from build123d import *

# Parameters (mm, degrees)
SKETCH3_R               = 3
CUT_EXTRUDE1_DEPTH      = 75.457245764
SKETCH4_R               = 41.3
SKETCH4_R_2             = 38
SKETCH4_R_3             = 3
CUT_EXTRUDE2_DEPTH      = 10
BOSS_EXTRUDE1_START     = -2
BOSS_EXTRUDE1_OUTLINE_R = 41.3
BOSS_EXTRUDE1_DEPTH     = 2
SKETCH5_R               = 3
SKETCH5_R_2             = 1.7
BOSS_EXTRUDE2_DEPTH     = 2


# Read off the part's stored shape, not the designer's step: Boss-Extrude1
with BuildPart() as part:
    # Sketch2 → Revolve1 (revolve)
    with BuildSketch(Plane(origin=(0, 0, 0), x_dir=(1, 0, 0), z_dir=(0, 1, 0)), mode=Mode.PRIVATE) as revolve1_sk:
        Polygon((-21.165551628, 4), (-21.165551628, -4), (-9.945763659, -4), align=None)
    revolve(revolve1_sk.sketch.rotate(Axis((20.134448372, 0, 4), (0, 0, -1)), 180), axis=Axis((20.134448372, 0, 4), (0, 0, -1)))

    # Sketch3 → Cut-Extrude1 (cut, through all)
    with BuildSketch(Plane.XY.offset(4)):
        with Locations((20.134448372, 35.5)):
            Circle(SKETCH3_R)
        with Locations((55.634448372, 0)):
            Circle(SKETCH3_R)
        with Locations((20.134448372, -35.5)):
            Circle(SKETCH3_R)
        with Locations((-15.365551628, 0)):
            Circle(SKETCH3_R)
    extrude(amount=-CUT_EXTRUDE1_DEPTH, mode=Mode.SUBTRACT)

    # Sketch4 → Cut-Extrude2 (cut)
    # profile 1 of 4: a face of its own
    with BuildSketch(Plane.XY.offset(4)):
        with Locations((20.134448372, 0)):
            Circle(SKETCH4_R)
        with Locations((20.134448372, 0)):
            Circle(SKETCH4_R_2, mode=Mode.SUBTRACT)
        with Locations((55.634448372, 0)):
            Circle(SKETCH4_R_3, mode=Mode.SUBTRACT)
    # profile 2 of 4: a face of its own
    with BuildSketch(Plane.XY.offset(4)):
        with Locations((20.134448372, -35.5)):
            Circle(SKETCH4_R_3)
    # profile 3 of 4: a face of its own
    with BuildSketch(Plane.XY.offset(4)):
        with Locations((-15.365551628, 0)):
            Circle(SKETCH4_R_3)
    # profile 4 of 4: a face of its own
    with BuildSketch(Plane.XY.offset(4)):
        with Locations((20.134448372, 35.5)):
            Circle(SKETCH4_R_3)
    extrude(amount=-CUT_EXTRUDE2_DEPTH, mode=Mode.SUBTRACT)

    # Boss-Extrude1 outline → Boss-Extrude1 (add)
    with BuildSketch(Plane.XY.offset(4).offset(BOSS_EXTRUDE1_START)):
        with Locations((20.134448372, 0)):
            Circle(BOSS_EXTRUDE1_OUTLINE_R)
        with BuildLine():
            ThreePointArc((21.849721462, 37.961267606), (47.004506057, 26.870057685), (58.095715978, 1.71527309))
            ThreePointArc((58.095715978, 1.71527309), (58.634448372, 0), (58.095715978, -1.71527309))
            ThreePointArc((58.095715978, -1.71527309), (47.004506057, -26.870057685), (21.849721462, -37.961267606))
            ThreePointArc((21.849721462, -37.961267606), (20.134448372, -38.5), (18.419175282, -37.961267606))
            ThreePointArc((18.419175282, -37.961267606), (-6.735609313, -26.870057685), (-17.826819233, -1.71527309))
            ThreePointArc((-17.826819233, -1.71527309), (-18.365551628, 0), (-17.826819233, 1.71527309))
            ThreePointArc((-17.826819233, 1.71527309), (-6.735609313, 26.870057685), (18.419175282, 37.961267606))
            ThreePointArc((18.419175282, 37.961267606), (20.134448372, 38.5), (21.849721462, 37.961267606))
        make_face(mode=Mode.SUBTRACT)
    extrude(amount=BOSS_EXTRUDE1_DEPTH)

    # Sketch5 → Boss-Extrude2 (add)
    # profile 1 of 4: a face of its own
    with BuildSketch(Plane.XY.offset(4)):
        with Locations((20.134448372, -35.5)):
            Circle(SKETCH5_R)
        with Locations((20.134448372, -35.5)):
            Circle(SKETCH5_R_2, mode=Mode.SUBTRACT)
    # profile 2 of 4: a face of its own
    with BuildSketch(Plane.XY.offset(4)):
        with Locations((-15.365551628, 0)):
            Circle(SKETCH5_R)
        with Locations((-15.365551628, 0)):
            Circle(SKETCH5_R_2, mode=Mode.SUBTRACT)
    # profile 3 of 4: a face of its own
    with BuildSketch(Plane.XY.offset(4)):
        with Locations((20.134448372, 35.5)):
            Circle(SKETCH5_R)
        with Locations((20.134448372, 35.5)):
            Circle(SKETCH5_R_2, mode=Mode.SUBTRACT)
    # profile 4 of 4: a face of its own
    with BuildSketch(Plane.XY.offset(4)):
        with Locations((55.634448372, 0)):
            Circle(SKETCH5_R)
        with Locations((55.634448372, 0)):
            Circle(SKETCH5_R_2, mode=Mode.SUBTRACT)
    extrude(amount=-BOSS_EXTRUDE2_DEPTH)


solid = part.part
Here's how the part is built. I have some questions about the finished solid (model axes, mm). A direction names the side the tool comes from. Coordinates: 2 decimals unless noted, no trailing zeros. Order: outer loops, then holes, each group sorted by start corner. A loop starts at its lowest first (then second) coordinate and runs counter-clockwise, first axis right, second up.
Item 1: If we mould it in two halves opening along X, with no side actions, what happens to faces 4 (the face through (22.92, 36.61, 0.61)), 5 (the face through (47.28, 26.59, 0.2)), 6 (the face through (-7.01, -26.59, 0.2))? For each: +X half, -X half, draft (parallel to the pull), parting line (faces both ways), or undercut.
Result sheet:
face 4: undercut
face 5: +X half
face 6: -X half
Item 2: For P1, Ø4.5, axis at x = -15.37, y = 0, coming from the -Z side; P2, Ø3, axis at x = -3, z = 3, coming from the +Y side, each with a flat end and sliding along its axis, tell me the tip position at first contact or that it passes through.
Result sheet:
P1: stops at z = 2
P2: stops at y = 35.18
Item 3: If we section it at A-A on y = 0: List the corners of the cut face in (x, z) for me, plus the area to 3 significant figures.
Result sheet:
outline: (-21.17, 2) - (-17.07, 2) - (-17.07, 4) - (-21.17, 4) - close; (-13.67, 2) - (-12.37, 2) - (-12.37, 2.27) - (-9.95, 4) - (-13.67, 4) - close; (50.21, 4) - (52.63, 2.27) - (52.63, 2) - (53.93, 2) - (53.93, 4) - close; (57.33, 2) - (61.43, 2) - (61.43, 4) - (57.33, 4) - close
area: 25.8 mm2
Item 4: For faces 1 (the face through (56.749, -2.785, 0.607)), 2 (the face through (46.72, -27.15, 0.2)), 3 (the face through (-6.456, 27.147, 0.202)), which set-ups out of +Z, -Z, +X, -X, +Y, -Y let a thin tool reach every point of the face, with its end or its side?
Result sheet:
face 1: -Z
face 2: -Z, +X, -Y
face 3: -Z, -X, +Y
Item 5: I need wall thicknesses on line 1 (X direction, y = -21, z = -0.65); line 2 (Z direction, x = -15, y = 2.5); line 3 (Y direction, x = 14.5, z = 3.1). Which ranges of each line are inside material? Lowest first, please.
Result sheet:
line 1: x = -11.54 to -9.84, 50.11 to 51.8
line 2: z = 2 to 4
line 3: y = -40.91 to -30.83, 30.83 to 40.91
Item 6: If we section it at B-B on z = 0.2: List the corners of the cut face in (x, y) for me.
Result sheet:
outline: (-17.83, -1.72) arc R38 ccw to (18.42, -37.96) arc R3 cw to (17.14, -35.28) arc R35.41 cw to (-15.15, -2.99) arc R3 cw to start; (-17.83, 1.72) arc R3 cw to (-15.15, 2.99) arc R35.41 cw to (17.14, 35.28) arc R3 cw to (18.42, 37.96) arc R38 ccw to start; (21.85, -37.96) arc R38 ccw to (58.1, -1.72) arc R3 cw to (55.42, -2.99) arc R35.41 cw to (23.13, -35.28) arc R3 cw to start; (21.85, 37.96) arc R3 cw to (23.13, 35.28) arc R35.41 cw to (55.42, 2.99) arc R3 cw to (58.1, 1.72) arc R38 ccw to start
